Here's how the part is built. I have some questions about the finished solid (model axes, mm). Face numbers are marked on the shaded views. A direction names the side the tool comes from. Give positions to 0.01 mm unless a question says otherwise; leave off trailing zeros. Loops run counter-clockwise (first coordinate to the right, second up) from the corner with the lowest first, then second, coordinate; pieces in that order, holes last. Notation, with made-up numbers: (1.5, -40) - (9.5, -40) arc R20 cw to (9.5, -18) - close; hole circle Ø5 at (-6, -23). An arc over 180 degrees is marked (long way). Use a Markdown table: item, result.
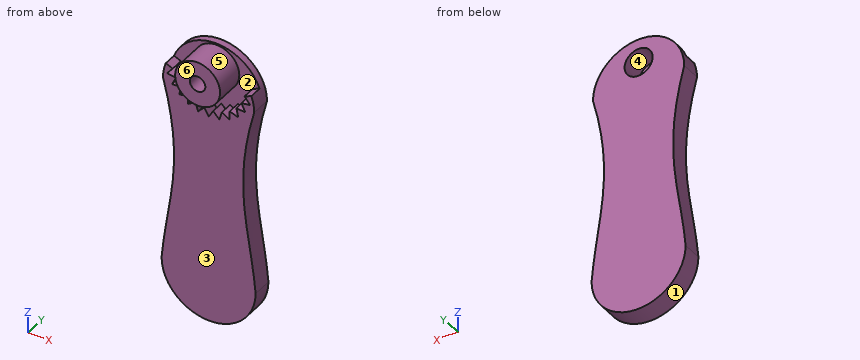
from build123d import *

# Parameters (mm, degrees)
F1_DEPTH = 7.112
F2_R     = 8.128
F2_R_2   = 2.794
F3_DEPTH = 6.096
F4_DEPTH = 50.8
F5_R     = 8.128
F6_DEPTH = 4.572
F7_R     = 5.08
F7_R_2   = 2.794
F8_DEPTH = 8.128


with BuildPart() as f1:
    # F0 (on Front) → F1 (new body)
    with BuildSketch(Plane.XZ):
        with BuildLine():
            add(Edge.make_bspline(
                [(16.51, 16.2022389048), (8.1950903917, -14.7107664531), (15.1309384414, -29.2677398155), (17.018, -51.8697610952)],
                knots=[0, 0, 0, 0, 68.073895496, 68.073895496, 68.073895496, 68.073895496], degree=3))
            ThreePointArc((16.51, 16.2022389048), (0, 32.7122389048), (-16.51, 16.2022389048))
            add(Edge.make_bspline(
                [(-16.51, 16.2022389048), (-8.1950903917, -14.7107664531), (-15.1309384414, -29.2677398155), (-17.018, -51.8697610952)],
                knots=[0, 0, 0, 0, 68.073895496, 68.073895496, 68.073895496, 68.073895496], degree=3))
            ThreePointArc((-17.018, -51.8697610952), (0, -68.8877610952), (17.018, -51.8697610952))
        make_face()
    extrude(amount=F1_DEPTH)

    # F2 (on face) → F3 (join)
    with BuildSketch(Plane.XZ.offset(7.112)):
        with Locations((0, 24.0762389048)):
            Circle(F2_R)
        with Locations((0, 24.0762389048)):
            Circle(F2_R_2, mode=Mode.SUBTRACT)
    extrude(amount=F3_DEPTH)

    # F4 (cut, symmetric): a face of the model
    f4_faces = [f1.faces().sort_by_distance(p)[0] for p in [
        (0, -7.112, 24.0762389048),
    ]]
    extrude(f4_faces, amount=F4_DEPTH, both=True, mode=Mode.SUBTRACT)

    # F5 (on face) → F6 (cut)
    with BuildSketch(Plane.XZ.offset(7.112)):
        with BuildLine():
            ThreePointArc((15.469928865, 21.9695087018), (-0.0442530739, 32.7121795972), (-15.5006234178, 21.8864955545))
            Line((-15.5006234178, 21.8864955545), (-12.9936152173, 20.8281131752))
            Line((-12.9936152173, 20.8281131752), (-15.0273981388, 18.3203464733))
            Line((-15.0273981388, 18.3203464733), (-11.8387170074, 17.8129221485))
            Line((-11.8387170074, 17.8129221485), (-13.2132540393, 14.8913104783))
            Line((-13.2132540393, 14.8913104783), (-9.995795597, 15.1617323254))
            Line((-9.995795597, 15.1617323254), (-10.6312036432, 11.9960691377))
            Line((-10.6312036432, 11.9960691377), (-7.5719548797, 13.0286212217))
            Line((-7.5719548797, 13.0286212217), (-7.4313063342, 9.8028833542))
            Line((-7.4313063342, 9.8028833542), (-4.7080596678, 11.5375575014))
            Line((-4.7080596678, 11.5375575014), (-3.7995285128, 8.4392131139))
            Line((-3.7995285128, 8.4392131139), (-1.570549141, 10.7751963679))
            Line((-1.570549141, 10.7751963679), (0.0530640951, 7.9843099742))
            Line((0.0530640951, 7.9843099742), (1.6582359931, 10.7858434794))
            Line((1.6582359931, 10.7858434794), (3.9025728106, 8.4646112522))
            Line((3.9025728106, 8.4646112522), (4.7906504787, 11.5688800644))
            Line((4.7906504787, 11.5688800644), (7.5252781797, 9.8522035834))
            Line((7.5252781797, 9.8522035834), (7.6446497718, 13.0787988828))
            Line((7.6446497718, 13.0787988828), (10.7106417342, 12.0664451452))
            Line((10.7106417342, 12.0664451452), (10.0543698074, 15.2278489412))
            Line((10.0543698074, 15.2278489412), (13.2735417227, 14.9786522665))
            Line((13.2735417227, 14.9786522665), (11.8797664159, 17.8911352617))
            Line((11.8797664159, 17.8911352617), (15.0650317137, 18.4195780548))
            Line((15.0650317137, 18.4195780548), (13.0147541814, 20.913877324))
            Line((13.0147541814, 20.913877324), (15.469928865, 21.9695087018))
        make_face()
        with BuildLine():
            Line((-11.7664292563, 17.8014187834), (-11.8387170074, 17.8129221485))
            Line((-11.8387170074, 17.8129221485), (-11.8075561021, 17.8791554056))
            ThreePointArc((-11.8075561021, 17.8791554056), (-11.7870567643, 17.84025319), (-11.7664292563, 17.8014187834))
        make_face(mode=Mode.SUBTRACT)
        with BuildLine():
            Line((-9.9228554611, 15.1678628183), (-9.995795597, 15.1617323254))
            Line((-9.995795597, 15.1617323254), (-9.9813908269, 15.2334982572))
            ThreePointArc((-9.9813908269, 15.2334982572), (-9.952177253, 15.2006322819), (-9.9228554611, 15.1678628183))
        make_face(mode=Mode.SUBTRACT)
        with BuildLine():
            Line((-12.9261809524, 20.7996444858), (-12.9936152173, 20.8281131752))
            Line((-12.9936152173, 20.8281131752), (-12.9475091354, 20.8849645215))
            ThreePointArc((-12.9475091354, 20.8849645215), (-12.9369153807, 20.842286921), (-12.9261809524, 20.7996444858))
        make_face(mode=Mode.SUBTRACT)
        with BuildLine():
            Line((-7.5026013746, 13.0520292908), (-7.5719548797, 13.0286212217))
            Line((-7.5719548797, 13.0286212217), (-7.5751433977, 13.1017490531))
            ThreePointArc((-7.5751433977, 13.1017490531), (-7.5389133745, 13.0768293692), (-7.5026013746, 13.0520292908))
        make_face(mode=Mode.SUBTRACT)
        with BuildLine():
            Line((-4.646323367, 11.5768827546), (-4.7080596678, 11.5375575014))
            Line((-4.7080596678, 11.5375575014), (-4.7286561687, 11.6077973086))
            ThreePointArc((-4.7286561687, 11.6077973086), (-4.6875152535, 11.5922721575), (-4.646323367, 11.5768827546))
        make_face(mode=Mode.SUBTRACT)
        with BuildLine():
            Line((-1.5200179341, 10.8281533646), (-1.570549141, 10.7751963679))
            Line((-1.570549141, 10.7751963679), (-1.6073566312, 10.8384660687))
            ThreePointArc((-1.6073566312, 10.8384660687), (-1.5636957843, 10.8332377157), (-1.5200179341, 10.8281533646))
        make_face(mode=Mode.SUBTRACT)
        with BuildLine():
            Line((1.6946254161, 10.8493545514), (1.6582359931, 10.7858434794))
            Line((1.6582359931, 10.7858434794), (1.6073566312, 10.8384660687))
            ThreePointArc((1.6073566312, 10.8384660687), (1.651, 10.8438383667), (1.6946254161, 10.8493545514))
        make_face(mode=Mode.SUBTRACT)
        with BuildLine():
            Line((4.8107832969, 11.639254179), (4.7906504787, 11.5688800644))
            Line((4.7906504787, 11.5688800644), (4.7286561687, 11.6077973086))
            ThreePointArc((4.7286561687, 11.6077973086), (4.7697456655, 11.6234580392), (4.8107832969, 11.639254179))
        make_face(mode=Mode.SUBTRACT)
        with BuildLine():
            Line((7.6473559389, 13.1519461522), (7.6446497718, 13.0787988828))
            Line((7.6446497718, 13.0787988828), (7.5751433977, 13.1017490531))
            ThreePointArc((7.5751433977, 13.1017490531), (7.6112910502, 13.1267880715), (7.6473559389, 13.1519461522))
        make_face(mode=Mode.SUBTRACT)
        with Locations((0, 24.0762389048)):
            Circle(F5_R, mode=Mode.SUBTRACT)
        with BuildLine():
            Line((11.8481693767, 17.9571615707), (11.8797664159, 17.8911352617))
            Line((11.8797664159, 17.8911352617), (11.8075561021, 17.8791554056))
            ThreePointArc((11.8075561021, 17.8791554056), (11.8279270467, 17.9181250071), (11.8481693767, 17.9571615707))
        make_face(mode=Mode.SUBTRACT)
        with BuildLine():
            Line((12.9682741648, 20.9704233621), (13.0147541814, 20.913877324))
            Line((13.0147541814, 20.913877324), (12.9475091354, 20.8849645215))
            ThreePointArc((12.9475091354, 20.8849645215), (12.9579621013, 20.9276768234), (12.9682741648, 20.9704233621))
        make_face(mode=Mode.SUBTRACT)
        with BuildLine():
            Line((-12.9475091354, 20.8849645215), (-12.9936152173, 20.8281131752))
            Line((-12.9936152173, 20.8281131752), (-12.9261809524, 20.7996444858))
            ThreePointArc((-12.9261809524, 20.7996444858), (-12.9369153807, 20.842286921), (-12.9475091354, 20.8849645215))
        make_face()
        with BuildLine():
            Line((-11.8075561021, 17.8791554056), (-11.8387170074, 17.8129221485))
            Line((-11.8387170074, 17.8129221485), (-11.7664292563, 17.8014187834))
            ThreePointArc((-11.7664292563, 17.8014187834), (-11.7870567643, 17.84025319), (-11.8075561021, 17.8791554056))
        make_face()
        with BuildLine():
            Line((-9.9813908269, 15.2334982572), (-9.995795597, 15.1617323254))
            Line((-9.995795597, 15.1617323254), (-9.9228554611, 15.1678628183))
            ThreePointArc((-9.9228554611, 15.1678628183), (-9.952177253, 15.2006322819), (-9.9813908269, 15.2334982572))
        make_face()
        with BuildLine():
            Line((-7.5751433977, 13.1017490531), (-7.5719548797, 13.0286212217))
            Line((-7.5719548797, 13.0286212217), (-7.5026013746, 13.0520292908))
            ThreePointArc((-7.5026013746, 13.0520292908), (-7.5389133745, 13.0768293692), (-7.5751433977, 13.1017490531))
        make_face()
        with BuildLine():
            Line((-4.7286561687, 11.6077973086), (-4.7080596678, 11.5375575014))
            Line((-4.7080596678, 11.5375575014), (-4.646323367, 11.5768827546))
            ThreePointArc((-4.646323367, 11.5768827546), (-4.6875152535, 11.5922721575), (-4.7286561687, 11.6077973086))
        make_face()
        with BuildLine():
            Line((-1.6073566312, 10.8384660687), (-1.570549141, 10.7751963679))
            Line((-1.570549141, 10.7751963679), (-1.5200179341, 10.8281533646))
            ThreePointArc((-1.5200179341, 10.8281533646), (-1.5636957843, 10.8332377157), (-1.6073566312, 10.8384660687))
        make_face()
        with BuildLine():
            Line((1.6073566312, 10.8384660687), (1.6582359931, 10.7858434794))
            Line((1.6582359931, 10.7858434794), (1.6946254161, 10.8493545514))
            ThreePointArc((1.6946254161, 10.8493545514), (1.651, 10.8438383667), (1.6073566312, 10.8384660687))
        make_face()
        with BuildLine():
            Line((4.7286561687, 11.6077973086), (4.7906504787, 11.5688800644))
            Line((4.7906504787, 11.5688800644), (4.8107832969, 11.639254179))
            ThreePointArc((4.8107832969, 11.639254179), (4.7697456655, 11.6234580392), (4.7286561687, 11.6077973086))
        make_face()
        with BuildLine():
            Line((7.5751433977, 13.1017490531), (7.6446497718, 13.0787988828))
            Line((7.6446497718, 13.0787988828), (7.6473559389, 13.1519461522))
            ThreePointArc((7.6473559389, 13.1519461522), (7.6112910502, 13.1267880715), (7.5751433977, 13.1017490531))
        make_face()
        with BuildLine():
            Line((11.8075561021, 17.8791554056), (11.8797664159, 17.8911352617))
            Line((11.8797664159, 17.8911352617), (11.8481693767, 17.9571615707))
            ThreePointArc((11.8481693767, 17.9571615707), (11.8279270467, 17.9181250071), (11.8075561021, 17.8791554056))
        make_face()
        with BuildLine():
            Line((12.9475091354, 20.8849645215), (13.0147541814, 20.913877324))
            Line((13.0147541814, 20.913877324), (12.9682741648, 20.9704233621))
            ThreePointArc((12.9682741648, 20.9704233621), (12.9579621013, 20.9276768234), (12.9475091354, 20.8849645215))
        make_face()
    extrude(amount=-F6_DEPTH, mode=Mode.SUBTRACT)

    # F7 (on face) → F8 (cut)
    with BuildSketch(Plane(origin=(0, 0, 0), x_dir=(-1, 0, 0), z_dir=(0, 1, 0))):
        with Locations((0, 24.0762389048)):
            Circle(F7_R)
        with Locations((0, 24.0762389048)):
            Circle(F7_R_2, mode=Mode.SUBTRACT)
    extrude(amount=-F8_DEPTH, mode=Mode.SUBTRACT)


solid = f1.part
(1) On a 3-axis mill with a long thin cutter (end or side, diameter ignored), from which of +Z, -Z, +X, -X, +Y, -Y can I reach the whole of each face in a straight line? I mean the marked faces 4, 5 and 6. Say none if no direction works.
A:
| item | result |
|---|---|
| face 4 | +Y |
| face 5 | -Y |
| face 6 | +Z, -Z, +X, -X, -Y |
(2) Suppose I cut it at B-B on z = -59.5. Write out the boundary of the cut face in (x, y), plus the area to 3 significant figures.
A:
| item | result |
|---|---|
| outline | (-15.21, -7.11) - (15.21, -7.11) - (15.21, 0) - (-15.21, 0) - close |
| area | 216 mm2 |
(3) Suppose I cut it at A-A on y = -9.75. Write out the boundary of the cut face in (x, z).
A:
| item | result |
|---|---|
| outline | circle Ø16.26 at (0, 24.08); hole circle Ø5.59 at (0, 24.08) |
(4) We'd pull the mould along X, two halves only. Please class the marked faces 1, 2 and 3: pulls with the +X half, pulls with the -X half, needs draft (parallel to the pull), parting line crosses it, or undercut.
A:
| item | result |
|---|---|
| face 1 | parting line crosses it |
| face 2 | undercut |
| face 3 | needs draft |
(5) If I drill on line 1 (Z direction, x = 0, y = -10.4); line 2 (Z direction, x = -1.5, y = -2.75); line 3 (Z direction, x = 0, y = -3.5), over which ranges is the centre line in solid material (lowest first)?
A:
| item | result |
|---|---|
| line 1 | 15.95 to 21.28, 26.87 to 32.2 |
| line 2 | -68.82 to 10.65, 16.09 to 19.22, 28.93 to 32.06 |
| line 3 | -68.89 to 8.08, 15.95 to 19, 29.16 to 32.2 |
(6) Will these pins go through, and if not, where does the flat tip stop? pin 1 (7.5 mm diameter, centred on x = 0, z = 24.08, fed in from -Y); pin 2 (1 mm diameter, centred on x = -2, y = -2.5, fed in from -Z); pin 3 (6 mm diameter, centred on y = -6, z = -12.5, fed in from +X); pin 4 (8 mm diameter, centred on x = -2, z = -38, fed in from -Y).
A:
| item | result |
|---|---|
| pin 1 | y = -13.21 |
| pin 2 | z = -68.82 |
| pin 3 | x = 12.58 |
| pin 4 | y = -7.11 |
